The listing builds one solid part. Answer for the finished solid, in the listing's coordinates (mm). A direction names the side the tool comes from. Give positions to 0.01 mm unless a question says otherwise; leave off trailing zeros. Loops run counter-clockwise (first coordinate to the right, second up) from the corner with the lowest first, then second, coordinate; pieces in that order, holes last.
Item 1: Each of these flat-tipped pins is pushed along its axis until it touches: pin 1 Ø0.5 at (y, z) = (1, 0.5) entering from +X; pin 2 Ø0.8 at (x, y) = (-21.5, 1) entering from +Z; pin 3 Ø0.5 at (x, y) = (21.5, 0.5) entering from -Z. Where does it stop, or does it pass through?
Item 2: Section A-A, the plane x = -17 is taken. Give the vertices of the cut face in (y, z), and give its area (3 significant figures).
Item 3: Section D-D, the plane x = 6.5 is taken. Give the vertices of the cut face in (y, z), and give its area (3 significant figures).
Item 4: A tool of negligible diameter and unlimited length cuts with its end or side. For faces 5 (the face through (21, 1, -0.8)), 6 (the face through (0, 1.6, 0)), 7 (the face through (0, 1, -15.98)), 8 (the face through (-21, 1, 0.8)), 9 (the face through (-0.8, 1, 21)), from which of +Z, -Z, +X, -X, +Y, -Y can it reach the whole face along a straight path? Write none if from no direction.
Item 5: Section C-C, the plane y = 0.45 is taken. Give the vertices of the cut face in (x, z).
Item 6: The mould has two halves that part along X. Classify faces 1 (the face through (15.98, 1, 0)), 2 (the face through (0.8, 1, -21)), 3 (the face through (-15.98, 1, 0)), 4 (the face through (0.8, 1, 21)): pulls with the +X half, pulls with the -X half, needs draft (parallel to the pull), parting line crosses it, or undercut.
Item 7: Section B-B, the plane z = 22.5 is taken. Give the vertices of the cut face in (x, y).
Item 8: Consider line 1 along Z through (x, y) = (0.5, 1.2); line 2 along X through (y, z) = (0.3, -19); line 3 along X through (y, z) = (0.6, -18.5). Determine where each line is inside the solid, lowest interval first.
Autodesk Inventor part; units mm, degrees
ref_plane "YZ Plane" through (0, 0, 0) normal (1, 0, 0) x (0, 1, 0)
ref_plane "XZ Plane" through (0, 0, 0) normal (0, 1, 0) x (-1, 0, 0)
ref_plane "XY Plane" through (0, 0, 0) normal (0, 0, 1) x (1, 0, 0)
sketch "Sketch1" plane through (0, 0, 0) normal (0, 1, 0) x (-1, 0, 0)
  point P0 (0, 0)
sketch "Sketch2" plane through (0, 0, 0) normal (0, 1, 0) x (-1, 0, 0)
  line L0 (46.5779, 0.8) -> (15.98, 0.8) construction
  line L1 (47.5028, -0.8) -> (-15.98, -0.8) construction
  line L2 (0.8, 38.8593) -> (0.8, 25.9877) construction
  line L3 (-0.8, 36.7319) -> (-0.8, -46.7895) construction
  arc A0 (15.98, 0.8) -> (0.8, 15.98) centre (0, 0) ccw construction
  arc A1 (-0.8, 15.98) -> (-15.98, 0.8) centre (0, 0) ccw construction
  line L4 (0.8, 25.9877) -> (0.8, -15.98) construction
  arc A2 (-0.8, 25.9877) -> (-25.9877, 0.8) centre (0, 0) ccw
  line L5 (0.8, -15.98) -> (0.8, -47.3445) construction
  arc A3 (0.8, -25.9877) -> (25.9877, -0.8) centre (0, 0) ccw
  arc A4 (25.9877, 0.8) -> (0.8, 25.9877) centre (0, 0) ccw
  line L6 (15.98, 0.8) -> (-25.9877, 0.8) construction
  line L7 (-15.98, -0.8) -> (-25.9877, -0.8) construction
  line L8 (-25.9877, 0.8) -> (-44.4844, 0.8) construction
  line L9 (-25.9877, -0.8) -> (-44.0655, -0.8) construction
  arc A5 (-25.9877, -0.8) -> (-0.8, -25.9877) centre (0, 0) ccw
  arc A6 (-15.98, -0.8) -> (-0.8, -15.98) centre (0, 0) ccw construction
  arc A7 (0.8, -15.98) -> (15.98, -0.8) centre (0, 0) ccw construction
  circle A8 centre (0, 0) radius 16 construction
  circle A9 centre (0, 0) radius 26 construction
  line L10 (25.9877, -0.8) -> (15.98, -0.8)
  line L11 (15.98, -0.8) -> (15.98, 0.8)
  line L12 (15.98, 0.8) -> (25.9877, 0.8)
  line L13 (0.8, -25.9877) -> (0.8, -15.98)
  line L14 (0.8, -15.98) -> (-0.8, -15.98)
  line L15 (-0.8, -15.98) -> (-0.8, -25.9877)
  line L16 (-25.9877, -0.8) -> (-15.98, -0.8)
  line L17 (-15.98, -0.8) -> (-15.98, 0.8)
  line L18 (-15.98, 0.8) -> (-25.9877, 0.8)
  line L19 (-0.8, 25.9877) -> (-0.8, 15.98)
  line L20 (-0.8, 15.98) -> (0.8, 15.98)
  line L21 (0.8, 15.98) -> (0.8, 25.9877)
  line L22 (0, 0) -> (-0.8, -25.9877) construction
  line L23 (0, 0) -> (-25.9877, -0.8) construction
  dimension "d2" = 0.8
  dimension "d3" = 0.8
  dimension "d4" = 0.8
  dimension "d5" = 0.8
  dimension "d6" = 32
  dimension "d7" = 0
  dimension "d8" = 0
  dimension "d9" = 52
  dimension "d10" = 0
  dimension "d11" = 0
  dimension "d12" = 0
  dimension "d15" = 86.474
extrude "Extrusion1" add sketch "Sketch2" along normal blind 1.6
properties part number "standin_quad_hub"
Worked answers:
1. pin 1: stops at x = 15.98
1. pin 2: stops at z = 15.19
1. pin 3: stops at z = -14.98
2. outline: (0, -19.67) - (1.6, -19.67) - (1.6, -0.8) - (0, -0.8) - close; (0, 0.8) - (1.6, 0.8) - (1.6, 19.67) - (0, 19.67) - close
2. area: 60.4 mm2
3. outline: (0, -25.17) - (1.6, -25.17) - (1.6, 25.17) - (0, 25.17) - close
3. area: 80.6 mm2
4. face 5: +X, +Y, -Y
4. face 6: +Z, -Z, +X, -X, +Y
4. face 7: -Z, +Y, -Y
4. face 8: -X, +Y, -Y
4. face 9: +Z, +Y, -Y
5. outline: (-25.99, -0.8) arc R26 ccw to (-0.8, -25.99) - (-0.8, -15.98) - (0.8, -15.98) - (0.8, -25.99) arc R26 ccw to (25.99, -0.8) - (15.98, -0.8) - (15.98, 0.8) - (25.99, 0.8) arc R26 ccw to (0.8, 25.99) - (0.8, 15.98) - (-0.8, 15.98) - (-0.8, 25.99) arc R26 ccw to (-25.99, 0.8) - (-15.98, 0.8) - (-15.98, -0.8) - close
6. face 1: pulls with the +X half
6. face 2: undercut
6. face 3: pulls with the -X half
6. face 4: undercut
7. outline: (-13.03, 0) - (-0.8, 0) - (-0.8, 1.6) - (-13.03, 1.6) - close; (0.8, 0) - (13.03, 0) - (13.03, 1.6) - (0.8, 1.6) - close
8. line 1: z = -15.98 to 15.98
8. line 2: x = -17.75 to -0.8, 0.8 to 17.75
8. line 3: x = -18.27 to -0.8, 0.8 to 18.27
